Model file for the job. Use its own axes, mm. A direction names the side the tool comes from. Give positions to 0.01 mm unless a question says otherwise; leave off trailing zeros. Write each loop counter-clockwise with the first axis right and the second up, starting at its lowest first coordinate (ties: lowest second). Pieces come first, ordered by that corner, then holes. Notation, with made-up numbers: (-18.75, 50.25) - (23.25, 50.25) arc R29 ccw to (23.25, 84.25) - close; hole circle Ø6 at (42.25, -9.75). An arc over 180 degrees is marked (long way). One line per item, written item: value. Start each with the question number.
(1) Cut at D-D, the plane z = 1. List the corners of the cut face in (x, y).
(2) Cut at C-C, the plane x = 0. List the corners of the cut face in (y, z).
(3) 3-axis set-ups, long thin cutter, end or side, ignore diameter. For faces 4 (the face through (14.1, 33, 7)), 5 (the face through (-17, 17, 15.1)), 6 (the face through (18, 7, 5.1)), 7 (the face through (-0.1, 3.5, -14.3)): which of +Z, -Z, +X, -X, +Y, -Y reach the whole face in a straight line?
(4) Cut at A-A, the plane z = 9.5. State how many separate pieces and enclosed holes the cut face has, and give its area (3 significant figures).
(5) Probe L1, parallel to Y at x = -17.6, z = 11; L2, parallel to Y at x = -4.5, z = -13.5; L3, parallel to X at y = 19, z = 8.5. List the from-to ranges inside material, lowest first.
(6) Drop flat-ended pins along their axis: P1, Ø12, axis at y = 9, z = -13, coming from the +X side; P2, Ø1.7, axis at x = -17.6, y = 28, coming from the +Z side; P3, Ø3, axis at x = -17.6, y = 21, coming from the -Z side. Give the stop position or say it passes through.
(7) Cut at B-B, the plane y = 16. List the corners of the cut face in (x, z).
(8) Mould opens along X. For faces 1 (the face through (3, 35, -14)), 2 (the face through (-20.1, 17, 7)), 3 (the face through (17.297, 19.633, 10.17)) say: pulls with the +X half, pulls with the -X half, needs draft (parallel to the pull), parting line crosses it, or undercut.
from build123d import *

# Parameters (mm, degrees)
BOSS_EXTRUDE1_DEPTH = 35
SKETCH2_W           = 30.2
SKETCH2_H           = 28
CUT_EXTRUDE1_DEPTH  = 54.554178175
BOSS_EXTRUDE2_START = -3.5
BOSS_EXTRUDE2_DEPTH = 3.5
BOSS_EXTRUDE3_DEPTH = 3.5
SKETCH6_R           = 1.4
CUT_EXTRUDE3_DEPTH  = 10


with BuildPart() as part:
    # Sketch1 → Boss-Extrude1 (new body)
    with BuildSketch(Plane(origin=(0, 0, 0), x_dir=(1, 0, 0), z_dir=(0, 1, 0))):
        with BuildLine():
            Line((15.1, 0), (15.1, -15.1))
            Line((15.1, -15.1), (20.1, -15.1))
            Line((20.1, -15.1), (20.1, 0))
            ThreePointArc((20.1, 0), (0, 20.1), (-20.1, 0))
            Line((-20.1, 0), (-20.1, -15.1))
            Line((-20.1, -15.1), (-15.1, -15.1))
            Line((-15.1, -15.1), (-15.1, 0))
            ThreePointArc((-15.1, 0), (0, 15.1), (15.1, 0))
        make_face()
    extrude(amount=BOSS_EXTRUDE1_DEPTH)

    # Sketch2 → Cut-Extrude1 (cut, through all)
    with BuildSketch(Plane.XY.offset(15.1)):
        with Locations((0, 17.5)):
            Rectangle(SKETCH2_W, SKETCH2_H)
    extrude(amount=-CUT_EXTRUDE1_DEPTH, mode=Mode.SUBTRACT)

    # Sketch3 → Boss-Extrude2 (add)
    with BuildSketch(Plane(origin=(0, 35, 0), x_dir=(1, 0, 0), z_dir=(0, 1, 0)).offset(BOSS_EXTRUDE2_START)):
        with BuildLine():
            Line((-15.1, 0), (-15.1, -15.1))
            Line((-15.1, -15.1), (-14.1, -15.1))
            Line((-14.1, -15.1), (-14.1, 0))
            ThreePointArc((-14.1, 0), (0, 14.1), (14.1, 0))
            Line((14.1, 0), (14.1, -15.1))
            Line((14.1, -15.1), (15.1, -15.1))
            Line((15.1, -15.1), (15.1, 0))
            ThreePointArc((15.1, 0), (0, 15.1), (-15.1, 0))
        make_face()
    extrude(amount=BOSS_EXTRUDE2_DEPTH)

    # Sketch4 → Boss-Extrude3 (add)
    with BuildSketch(Plane(origin=(0, 0, 0), x_dir=(-1, 0, 0), z_dir=(0, -1, 0))):
        with BuildLine():
            Line((15.1, 0), (15.1, -15.1))
            Line((15.1, -15.1), (14.1, -15.1))
            Line((14.1, -15.1), (14.1, 0))
            ThreePointArc((14.1, 0), (0, 14.1), (-14.1, 0))
            Line((-14.1, 0), (-14.1, -15.1))
            Line((-14.1, -15.1), (-15.1, -15.1))
            Line((-15.1, -15.1), (-15.1, 0))
            ThreePointArc((-15.1, 0), (0, 15.1), (15.1, 0))
        make_face()
    extrude(amount=-BOSS_EXTRUDE3_DEPTH)

    # Sketch6 → Cut-Extrude3 (cut)
    with BuildSketch(Plane.XY.offset(15.1)):
        with Locations((-17.6, 28)):
            Circle(SKETCH6_R)
        with Locations((17.6, 28)):
            Circle(SKETCH6_R)
        with Locations((17.6, 21)):
            Circle(SKETCH6_R)
        with Locations((17.6, 14)):
            Circle(SKETCH6_R)
        with Locations((17.6, 7)):
            Circle(SKETCH6_R)
        with Locations((-17.6, 21)):
            Circle(SKETCH6_R)
        with Locations((-17.6, 14)):
            Circle(SKETCH6_R)
        with Locations((-17.6, 7)):
            Circle(SKETCH6_R)
    extrude(amount=-CUT_EXTRUDE3_DEPTH, mode=Mode.SUBTRACT)


solid = part.part
Answers follow:
1. outline: (-20.1, 0) - (-14.1, 0) - (-14.1, 3.5) - (-15.1, 3.5) - (-15.1, 31.5) - (-14.1, 31.5) - (-14.1, 35) - (-20.1, 35) - close; (14.1, 0) - (20.1, 0) - (20.1, 35) - (14.1, 35) - (14.1, 31.5) - (15.1, 31.5) - (15.1, 3.5) - (14.1, 3.5) - close
2. outline: (0, -20.1) - (3.5, -20.1) - (3.5, -14.1) - (0, -14.1) - close; (31.5, -20.1) - (35, -20.1) - (35, -14.1) - (31.5, -14.1) - close
3. face 4: +Z, +Y, -Y
3. face 5: +Z, +X, -X, +Y, -Y
3. face 6: +Z
3. face 7: +Z, -Z
4. separate pieces: 2
4. enclosed holes: 8
4. area: 315 mm²
5. L1: y = 0 to 5.6, 8.4 to 12.6, 15.4 to 19.6, 22.4 to 26.6, 29.4 to 35
5. L2: y = 0 to 3.5, 31.5 to 35
5. L3: x = -20.1 to -15.1, 15.1 to 20.1
6. P1: stops at x = 18.84
6. P2: stops at z = 5.1
6. P3: stops at z = -12.03
7. outline: (-20.1, 0) arc R20.1 ccw to (-15.1, -13.27) - (-15.1, 15.1) - (-20.1, 15.1) - close; (15.1, -13.27) arc R20.1 ccw to (20.1, 0) - (20.1, 15.1) - (15.1, 15.1) - close
8. face 1: needs draft
8. face 2: pulls with the -X half
8. face 3: undercut
